The listing builds one solid part. Answer for the finished solid, in the listing's coordinates (mm). Coordinates: 2 decimals unless noted, no trailing zeros. Loops run counter-clockwise (first coordinate to the right, second up) from the corner with the lowest first, then second, coordinate; pieces in that order, holes last. Notation, with made-up numbers: (30.25, 58.25) - (41.25, 58.25) arc R21 ccw to (41.25, 78.25) - close; hole circle Ø10 at (46, 64.5). An arc over 180 degrees is marked (long way). Put each result on its own line as item: value.
```python
from build123d import *

# Parameters (mm, degrees)
BOSS_EXTRUDE1_DEPTH      = 19.05
BOSS_EXTRUDE1_DEPTH_BACK = 19.05
FILLET1_R                = 0.254


with BuildPart() as part:
    # Sketch1 → Boss-Extrude1 (new, two sides: drawn at the far end of the back side and taken through both)
    with BuildSketch(Plane.XY.offset(-BOSS_EXTRUDE1_DEPTH_BACK)):
        Polygon((388.793340161, 276.463831059), (354.511506684, 255.928673382), (354.511506684, 238.923904635), (402.896942526, 238.923904635), (424.852995025, 246.325755667), (417.308575132, 268.704709057), align=None)
    extrude(amount=BOSS_EXTRUDE1_DEPTH + BOSS_EXTRUDE1_DEPTH_BACK)

    # Fillet1
    fillet1_edges = [part.edges().sort_by_distance(p)[0] for p in [
        (371.652423423, 266.19625222, -19.05),
        (424.852995025, 246.325755667, 0),
        (402.896942526, 238.923904635, 0),
        (354.511506684, 238.923904635, 0),
        (354.511506684, 255.928673382, 0),
        (388.793340161, 276.463831059, 0),
        (417.308575132, 268.704709057, 0),
        (354.511506684, 247.426289008, -19.05),
        (378.704224605, 238.923904635, -19.05),
        (421.080785078, 257.515232362, 19.05),
        (403.050957647, 272.584270058, 19.05),
        (371.652423423, 266.19625222, 19.05),
        (354.511506684, 247.426289008, 19.05),
        (378.704224605, 238.923904635, 19.05),
        (413.874968775, 242.624830151, -19.05),
        (413.874968775, 242.624830151, 19.05),
        (421.080785078, 257.515232362, -19.05),
        (403.050957647, 272.584270058, -19.05),
    ]]
    fillet(fillet1_edges, radius=FILLET1_R)


solid = part.part
```
1) This flat-tipped pin is pushed along its axis until it touches: pin 1 (8 mm diameter, centred on y = 248.5, z = 12.5, fed in from +X). Where does it stop, or does it pass through?
Found:
pin 1: stops at x = 424.79
2) Straight lines are drawn through the part: L1, parallel to Y at x = 413.5, z = -10.5; L2, parallel to Y at x = 373, z = 6; L3, parallel to X at y = 267.5, z = 10. For each, find the intervals that lie inside material, in ascending order. Write a range as [from, to].
Found:
L1: y = [242.5, 269.74]
L2: y = [238.92, 267]
L3: x = [373.83, 417.71]
3) The part is cut by section A-A (z = -7). Give the vertices of the cut face in (x, y), and give its area (3 significant figures).
Found:
outline: (354.51, 239.18) arc R0.25 ccw to (354.77, 238.92) - (402.86, 238.92) arc R0.25 ccw to (402.94, 238.94) - (424.61, 246.24) arc R0.25 ccw to (424.77, 246.57) - (417.35, 268.58) arc R0.25 ccw to (417.18, 268.74) - (388.9, 276.44) arc R0.25 ccw to (388.7, 276.41) - (354.63, 256) arc R0.25 ccw to (354.51, 255.78) - close
area: 1,950 mm^2
